Here's the drawing with two shaded views (mm, measured from the low corner). I have some questions. Coordinates: 2 decimals unless noted, no trailing zeros. Write each loop counter-clockwise with the first axis right and the second up, starting at its lowest first coordinate (ties: lowest second). Pieces come first, ordered by that corner, then holes. Notation, with made-up numbers: (23, 10) -> (46, 10) arc R17 cw to (46, 24) -> close; hole circle Ø1 at (-9.75, -6.75). An arc over 180 degrees is marked (long way). Answer in a Markdown table with one row per item. Add a question column.
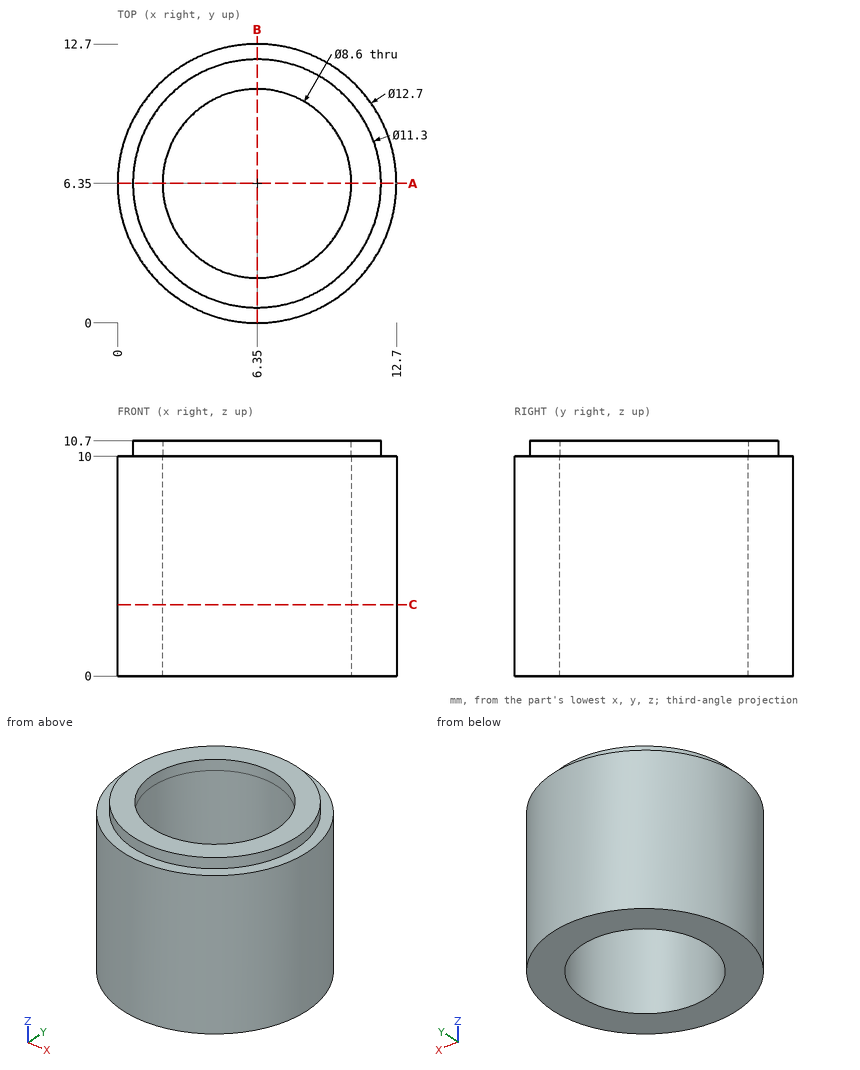
Q1. I need wall thicknesses on line 1 (Y direction, x = 6.35, z = 6.75); line 2 (X direction, y = 2.5, z = 3); line 3 (Y direction, x = 6.35, z = 10.5). Which ranges of each line are inside material? Lowest first, please. Write a range as [from, to].
Q2. Imagine slicing it at A-A on y = 6.35. Please give me the cut outline in (x, z), plus the area to 3 significant figures.
Q3. Imagine slicing it at C-C on z = 3.25. Please give me the cut outline in (x, y).
Q4. I'm going to push flat-ended pins straight in: P1, Ø6.5, axis at x = 8, y = 6.5, coming from the +Z side; P2, Ø4, axis at y = 11.5, z = 7, coming from the +X side; P3, Ø6, axis at x = 9.5, z = 4, coming from the +Y side; P4, Ø4, axis at x = 1.5, z = 7, coming from the -Y side. Where does each tip first touch, or does it pass through?
Result sheet:
| question | item | result |
|---|---|---|
| 1 | line 1 | y = [0, 2.05], [10.65, 12.7] |
| 1 | line 2 | x = [1.3, 4.43], [8.27, 11.4] |
| 1 | line 3 | y = [0.7, 2.05], [10.65, 12] |
| 2 | outline | (0, 0) -> (2.05, 0) -> (2.05, 10.7) -> (0.7, 10.7) -> (0.7, 10) -> (0, 10) -> close; (10.65, 0) -> (12.7, 0) -> (12.7, 10) -> (12, 10) -> (12, 10.7) -> (10.65, 10.7) -> close |
| 2 | area | 42.9 mm^2 |
| 3 | outline | circle Ø12.7 at (6.35, 6.35); hole circle Ø8.6 at (6.35, 6.35) |
| 4 | P1 | stops at z = 10.7 |
| 4 | P2 | stops at x = 11.86 |
| 4 | P3 | stops at y = 12.7 |
| 4 | P4 | stops at y = 0.68 |
